```python
from build123d import *

# Parameters (mm, degrees)
ESQUISSE1_W                 = 24
ESQUISSE1_H                 = 30
MAIN_EXTRUSION_DEPTH        = 30
MAIN_RIDING_HOLE_DEPTH      = 36.623026261
ESQUISSE4_R                 = 2.25
TRACTORHOLE_DEPTH           = 8
IMPACTPIECE_DEPTH           = 4.5
CONG_1_R                    = 3
TEETH_DEPTH                 = 4.5
CONG_3_R                    = 0.57
TEETHREPETITION_COUNT       = 8
TEETHREPETITION_PITCH       = 4.71238898
CONG_3_OF_TEETHREPETITION_R = 0.57
ESQUISSE9_W                 = 55
ESQUISSE9_H                 = 15.375
BRACKET_DEPTH               = 0.675
ESQUISSE10_R                = 1.6
BRACKETHOLE_DEPTH           = 60.348546739
BRACKETHOLEREPETITION_COUNT = 5
BRACKETHOLEREPETITION_PITCH = 10
ESQUISSE11_W                = 7.5
ESQUISSE11_H                = 5.5
ESQUISSE11_H_2              = 7.6
RAILHOLE_DEPTH              = 20
TOPIMPACTCUT_DEPTH          = 60.348546739
ESQUISSE13_W                = 24
ESQUISSE13_H                = 50
MAKERBEAMMAINHOLE_DEPTH     = 95.451045521
KEEPONLYTRACTOR1_DEPTH      = 77.295478241
SKETCH2_W                   = 20
SKETCH2_H                   = 5.6
KEEPONLYTRACTOR2_DEPTH      = 41.263670039


with BuildPart() as part:
    # Esquisse1 → Main Extrusion (new body)
    with BuildSketch(Plane.XY):
        Rectangle(ESQUISSE1_W, ESQUISSE1_H)
    extrude(amount=MAIN_EXTRUSION_DEPTH)

    # Esquisse3 → Main Riding Hole (cut, through all)
    with BuildSketch(Plane(origin=(0, 0, 0), x_dir=(-1, 0, 0), z_dir=(0, 0, -1))):
        Polygon((-5.2, -1.6), (-5.2, -5.4), (-4.2, -5.4), (-4.2, -8.2), (-5.2, -8.2), (-5.2, -12), (-1.4, -12), (-1.4, -11), (1.4, -11), (1.4, -12), (5.2, -12), (5.2, -8.2), (4.2, -8.2), (4.2, -5.4), (5.2, -5.4), (5.2, -1.6), (1.4, -1.6), (1.4, -2.6), (-1.4, -2.6), (-1.4, -1.6), align=None)
    extrude(amount=-MAIN_RIDING_HOLE_DEPTH, mode=Mode.SUBTRACT)

    # Esquisse4 → TractorHole (cut)
    with BuildSketch(Plane.ZY.offset(12)):
        with Locations(Location((5, -6.8, 0), (0, 0, 270))):
            Circle(ESQUISSE4_R)
    tractorhole = extrude(amount=-TRACTORHOLE_DEPTH, mode=Mode.SUBTRACT)

    # TractorHoleSymetry: TractorHole across plane
    add(tractorhole.mirror(Plane(origin=(0, 0, 0), x_dir=(0, 0, 1), z_dir=(1, 0, 0))), mode=Mode.SUBTRACT)

    # Esquisse5 → ImpactPiece (add, symmetric)
    with BuildSketch(Plane(origin=(0, 0, 0), x_dir=(0, 0, -1), z_dir=(1, 0, 0))):
        Polygon((-45, 5), (-45, 35), (-25, 35), (-21.473460386, 15), (35, 15), (35, 3), (0, 3), (0, 5), align=None)
    extrude(amount=IMPACTPIECE_DEPTH, both=True)

    # Congé1
    cong_1_edges = [part.edges().sort_by_distance(p)[0] for p in [
        (4.5, 15, 25.736730193),
        (-4.5, 15, 25.736730193),
    ]]
    fillet(cong_1_edges, radius=CONG_1_R)

    # Esquisse8 → Teeth (add, symmetric)
    with BuildSketch(Plane(origin=(0, 0, 0), x_dir=(0, 0, -1), z_dir=(1, 0, 0))):
        Polygon((30, 15), (31.228399541, 18.375), (32.492683328, 18.375), (33.721082869, 15), align=None)
    teeth = extrude(amount=TEETH_DEPTH, both=True)

    # Congé3
    cong_3_edges = [part.edges().sort_by_distance(p)[0] for p in [
        (0, 15, -30),
        (0, 15, -33.721082869),
    ]]
    fillet(cong_3_edges, radius=CONG_3_R)

    # TeethRepetition: Teeth ×8
    with Locations(*[(0, 0, i * TEETHREPETITION_PITCH) for i in range(1, TEETHREPETITION_COUNT)]):
        add(teeth)

    # Congé3 of TeethRepetition
    cong_3_of_teethrepetition_edges = [part.edges().sort_by_distance(p)[0] for p in [
        (0, 15, -25.28761102),
        (0, 15, -29.008693889),
        (0, 15, -20.57522204),
        (0, 15, -24.296304909),
        (0, 15, -15.86283306),
        (0, 15, -19.583915929),
        (0, 15, -11.15044408),
        (0, 15, -14.871526949),
        (0, 15, -6.4380551),
        (0, 15, -10.159137969),
        (0, 15, -1.72566612),
        (0, 15, -5.446748989),
        (0, 15, 2.98672286),
        (0, 15, -0.734360009),
    ]]
    fillet(cong_3_of_teethrepetition_edges, radius=CONG_3_OF_TEETHREPETITION_R)

    # Esquisse9 → Bracket (cut, symmetric)
    with BuildSketch(Plane(origin=(4.5, 0, 0), x_dir=(0, 0, -1), z_dir=(1, 0, 0))):
        with Locations((7.5, 10.6875)):
            Rectangle(ESQUISSE9_W, ESQUISSE9_H)
    bracket = extrude(amount=BRACKET_DEPTH, both=True, mode=Mode.SUBTRACT)

    # Esquisse10 → BracketHole (cut, symmetric)
    with BuildSketch(Plane.ZY.offset(-4.5)):
        with Locations((-27, 9.1)):
            Circle(ESQUISSE10_R)
    brackethole = extrude(amount=BRACKETHOLE_DEPTH, both=True, mode=Mode.SUBTRACT)

    # BracketHoleRepetition: BracketHole ×5
    with Locations(*[(0, 0, i * BRACKETHOLEREPETITION_PITCH) for i in range(1, BRACKETHOLEREPETITION_COUNT)]):
        add(brackethole, mode=Mode.SUBTRACT)

    # Symétrie1: Bracket across plane
    add(bracket.mirror(Plane(origin=(0, 0, 0), x_dir=(0, 0, 1), z_dir=(1, 0, 0))), mode=Mode.SUBTRACT)

    # Esquisse11 → RailHole (cut)
    with BuildSketch(Plane(origin=(0, 0, 0), x_dir=(-1, 0, 0), z_dir=(0, 0, -1))):
        with Locations((8.25, 3.15)):
            Rectangle(ESQUISSE11_W, ESQUISSE11_H)
        with Locations((8.25, 16.2)):
            Rectangle(ESQUISSE11_W, ESQUISSE11_H_2)
    extrude(amount=-RAILHOLE_DEPTH, mode=Mode.SUBTRACT)

    # Esquisse12 → TopImpactCut (cut, through all)
    with BuildSketch(Plane(origin=(4.5, 0, 0), x_dir=(0, 0, -1), z_dir=(1, 0, 0))):
        Polygon((-45, 30), (-40, 35), (-45, 35), align=None)
    extrude(amount=-TOPIMPACTCUT_DEPTH, mode=Mode.SUBTRACT)


with BuildPart() as body_2:
    # Symétrie2: mirrored copy
    add(part.part.mirror(Plane(origin=(12, 15, 30), x_dir=(0, 0, 1), z_dir=(-1, 0, 0))))

    # Sketch1 → KeepOnlyTractor1 (cut, through all)
    with BuildSketch(Plane(origin=(0, 35, 0), x_dir=(1, 0, 0), z_dir=(0, 1, 0))):
        Polygon((12, 0), (12, -45), (36, -45), (36, 0), (27.825, 0.05190699), (27.825, -20), (20.175, -20), (20.175, 0), align=None)
    extrude(amount=-KEEPONLYTRACTOR1_DEPTH, mode=Mode.SUBTRACT)


with BuildPart() as part_1:
    add(part.part)

    # Esquisse13 → MakerBeamMainHole (cut, through all)
    with BuildSketch(Plane(origin=(0, 0, -35), x_dir=(-1, 0, 0), z_dir=(0, 0, -1))):
        with Locations((0, 10)):
            Rectangle(ESQUISSE13_W, ESQUISSE13_H)
    extrude(amount=-MAKERBEAMMAINHOLE_DEPTH, mode=Mode.SUBTRACT)


with BuildPart() as keeponlytractor1_kept_piece:
    # of the separate pieces the step leaves, the one the design keeps (keeponlytractor1_pieces_kept)
    add(body_2.part.solids().sort_by_distance((27.825, 15, 3.385841157))[0])

    # Sketch2 → KeepOnlyTractor2 (cut, through all)
    with BuildSketch(Plane.ZY.offset(-20.175)):
        with Locations((10, 0.2)):
            Rectangle(SKETCH2_W, SKETCH2_H)
    extrude(amount=-KEEPONLYTRACTOR2_DEPTH, mode=Mode.SUBTRACT)


solid = keeponlytractor1_kept_piece.part
```
The model under review builds one solid part; all positions refer to its coordinate system, in mm. A direction names the side the tool comes from. Give positions to 0.01 mm unless a question says otherwise; leave off trailing zeros. Write each loop counter-clockwise with the first axis right and the second up, starting at its lowest first coordinate (ties: lowest second). Pieces come first, ordered by that corner, then holes. Notation, with made-up numbers: (67, -40) - (102, -40) arc R17 cw to (102, -13) - close; hole circle Ø4 at (62, -28.75). An arc over 180 degrees is marked (long way). Answer in a Markdown table with one row per item. Add a question column.
1. Tool access review of faces 1 (the flat face through (24, 3, -8)), 2 (the flat face through (24, 15, 12)), 3 (the flat face through (23.946, 16.896, -0.044)): name each direction out of +Z, -Z, +X, -X, +Y, -Y from which nothing blocks a thin tool from reaching the whole face with its end or side.
2. Wall thickness on line 1 along Y through (x, z) = (25.5, 13); line 2 along Y through (x, z) = (22.5, -27) (3 decimals); line 3 along Z through (x, y) = (27.25, 8.5): over which ranges is each line inside the solid? List them lowest first. Write a range as [from, to].
3. Draft analysis for pull direction Z (two halves, no side actions). For faces 4 (the flat face through (23.95, 16.85, -21.25)), 5 (the flat face through (23.946, 16.854, 2.312)), 6 (the flat face through (23.95, 16.9, -33.03)), 7 (the flat face through (27.825, 11, -7)), state which applies: +Z half, -Z half, draft (parallel to the pull), parting line (faces both ways), or undercut.
4. We need section C-C on y = 16.5. State how many separate pieces and enclosed holes the cut face has, then the cut area to 3 significant figures.
5. We need section A-A on z = 13. Write out the cut boundary in (x, y) (3 decimals), then the cut area to 3 significant figures.
6. We need section D-D on z = -27. Write out the cut boundary in (x, y) (3 decimals), then the cut area to 3 significant figures.
7. We need section B-B on y = 9.1. Write out the cut boundary in (x, z) (3 decimals).
8. Insertion check: P1, Ø3, axis at x = 24, z = -24, coming from the +Y side (3 decimals); P2, Ø2.5, axis at y = 9.1, z = -27, coming from the -X side. Each pin has a flat end and moves straight along its axis. Give the tip position at first contact, or say it passes through.
Ans:
| question | item | result |
|---|---|---|
| 1 | face 1 | +Z, -Z, +X, -X, -Y |
| 1 | face 2 | +Z, +X, -X, +Y |
| 1 | face 3 | +X, -X, +Y |
| 2 | line 1 | y = [3, 7.5], [10.7, 15] |
| 2 | line 2 | y = [3, 7.5], [10.7, 18.375] |
| 2 | line 3 | z = [-35, -28.48], [-25.52, -18.48], [-15.52, -8.48], [-5.52, 1.52], [4.48, 11.52], [14.48, 20] |
| 3 | face 4 | undercut |
| 3 | face 5 | +Z half |
| 3 | face 6 | -Z half |
| 3 | face 7 | draft |
| 4 | separate pieces | 8 |
| 4 | enclosed holes | 0 |
| 4 | area | 161 mm^2 |
| 5 | outline | (20.175, 3) - (27.825, 3) - (27.825, 7.5) - (20.175, 7.5) - close; (20.175, 10.7) - (27.825, 10.7) - (27.825, 15) - (20.175, 15) - close |
| 5 | area | 67.3 mm^2 |
| 6 | outline | (20.175, 3) - (27.825, 3) - (27.825, 7.5) - (20.175, 7.5) - close; (20.175, 10.7) - (27.825, 10.7) - (27.825, 18.375) - (20.175, 18.375) - close |
| 6 | area | 93.1 mm^2 |
| 7 | outline | (20.175, -35) - (27.825, -35) - (27.825, -28.6) - (20.175, -28.6) - close; (20.175, -25.4) - (27.825, -25.4) - (27.825, -18.6) - (20.175, -18.6) - close; (20.175, -15.4) - (27.825, -15.4) - (27.825, -8.6) - (20.175, -8.6) - close; (20.175, -5.4) - (27.825, -5.4) - (27.825, 1.4) - (20.175, 1.4) - close; (20.175, 4.6) - (27.825, 4.6) - (27.825, 11.4) - (20.175, 11.4) - close; (20.175, 14.6) - (27.825, 14.6) - (27.825, 20) - (20.175, 20) - close |
| 8 | P1 | stops at y = 18.375 |
| 8 | P2 | passes through |
